Verification items for the finished model (mm, model axes). A direction names the side the tool comes from. Give positions to 0.01 mm unless a question says otherwise; leave off trailing zeros. Order: outer loops, then holes, each group sorted by start corner. A loop starts at its lowest first (then second) coordinate and runs counter-clockwise, first axis right, second up. Notation, with made-up numbers: (10, 37.5) -> (29, 37.5) arc R16 cw to (29, 58.5) -> close; hole circle Ø7 at (64, 70). An arc over 180 degrees is marked (long way). Return JSON: item names as keys, results as strings. Group by question number.
(1) Tool access check on faces 1 (the face through (5.08, 28, 3)), 2 (the face through (0, 28, 4.245)), 3 (the face through (4, 1, 2.54)). Record the directions out of +Z, -Z, +X, -X, +Y, -Y that give a thin tool (end or side, any length) a straight path to the whole face; none if there is none.
(2) Release check for a two-part mould opening along X. For faces 4 (the face through (3.726, 0, 4)), 5 (the face through (-2.961, 1, 4)), 6 (the face through (-8.69, 0, 3)), 7 (the face through (0, 28, 1.705)) record: pulls with the +X half, pulls with the -X half, needs draft (parallel to the pull), parting line crosses it, or undercut.
(3) Cross-section at C-C on x = -7.5. Enter the section's corners in (y, z), then the cut area to 3 significant figures.
(4) Thickness scan on line 1 along Y through (x, z) = (0.25, 2.8); line 2 along X through (y, z) = (7.5, 3.65); line 3 along Y through (x, z) = (-8, 4.9). Record the ranges inside material, lowest first.
(5) Cross-section at B-B on z = 1.05. Enter the section's corners in (x, y).
(6) Depth check by flat-ended pin: pin 1 Ø0.8 at (y, z) = (26, 3) entering from -X; pin 2 Ø1.5 at (x, z) = (-6.5, 2.5) entering from +Y; pin 3 Ø4 at (x, y) = (-2, 27.5) entering from -Z (3 decimals). Enter the tip coordinate at first touch or a pass-through.
(7) Cross-section at A-A on z = 3.1. State how many separate pieces and enclosed holes the cut face has, then the cut area to 3 significant figures.
from build123d import *

# Parameters (mm, degrees)
SKETCH1_W           = 17.38
SKETCH1_H           = 47.498
BOSS_EXTRUDE1_DEPTH = 5.95
CUT_EXTRUDE1_DEPTH  = 3.41
SKETCH3_W           = 10.16
SKETCH3_H           = 2.54
BOSS_EXTRUDE2_DEPTH = 7.62


with BuildPart() as part:
    # Sketch1 → Boss-Extrude1 (new body)
    with BuildSketch(Plane.XY):
        Rectangle(SKETCH1_W, SKETCH1_H)
    extrude(amount=BOSS_EXTRUDE1_DEPTH)

    # Sketch2 → Cut-Extrude1 (cut)
    with BuildSketch(Plane.XY.offset(5.95)):
        with BuildLine():
            add(Edge.make_bspline(
                [(0.550302732, -8.226542522), (0.379735674, -8.222982783), (0.040169774, -8.215896034), (-0.463839474, -8.15812923), (-0.957953156, -8.065305599), (-1.440722609, -7.93397308), (-1.914246856, -7.765779149), (-2.375520379, -7.555268135), (-2.829688826, -7.311649662), (-3.271985998, -7.033523648), (-3.695622296, -6.719710376), (-4.100608986, -6.379462985), (-4.482356898, -6.010283848), (-4.834867943, -5.609039062), (-5.170252218, -5.186152795), (-5.479691278, -4.732982281), (-5.767177385, -4.252361088), (-6.026195622, -3.745122286), (-6.262649235, -3.220813492), (-6.463385677, -2.677755241), (-6.63458604, -2.121971034), (-6.777705411, -1.554373675), (-6.884857685, -0.974513718), (-6.963012588, -0.382925268), (-7.013958172, 0.222378933), (-7.018848737, 0.631170896), (-7.021320272, 0.837761211)],
                knots=[0, 0, 0, 0, 0.935229359, 1.861860104, 2.778365642, 3.690213086, 4.602953262, 5.531139642, 6.468158725, 7.427752723, 8.393775505, 9.35721743, 10.326918663, 11.30305363, 12.284324182, 13.285316018, 14.310199044, 15.353667505, 16.407211588, 17.462763663, 18.526572315, 19.595421863, 20.671172186, 21.758519085, 22.867227609, 24, 24, 24, 24], degree=3))
            add(Edge.make_bspline(
                [(-7.021320272, 0.837761211), (-7.019018375, 1.043132905), (-7.014463737, 1.449490733), (-6.960970524, 2.051780421), (-6.891552806, 2.643471616), (-6.774881724, 3.22130983), (-6.639867653, 3.790672361), (-6.466996952, 4.345851556), (-6.265031095, 4.888970049), (-6.033789785, 5.416782083), (-5.779586146, 5.927183042), (-5.493336967, 6.408001352), (-5.191668967, 6.865492143), (-4.867252969, 7.295030074), (-4.519766848, 7.695667308), (-4.148181052, 8.065835718), (-3.757073623, 8.410721014), (-3.34206406, 8.721642737), (-2.915815576, 9.008687913), (-2.469246401, 9.247584189), (-2.017296753, 9.462224383), (-1.549212621, 9.625945007), (-1.073318626, 9.765137224), (-0.584345141, 9.855228751), (-0.084297826, 9.914279226), (0.252836758, 9.921036178), (0.42342487, 9.924455156)],
                knots=[0, 0, 0, 0, 1.133047579, 2.241899783, 3.335215261, 4.419027891, 5.492968413, 6.563480614, 7.625684211, 8.689373082, 9.742419676, 10.770259333, 11.775568516, 12.765501156, 13.738725683, 14.699866048, 15.658232057, 16.613840314, 17.560131627, 18.490982804, 19.406287858, 20.318317554, 21.224515383, 22.140052105, 23.058877329, 24, 24, 24, 24], degree=3))
            add(Edge.make_bspline(
                [(0.42342487, 9.924455156), (0.559148281, 9.921645508), (0.832560203, 9.915985532), (1.243556078, 9.86754079), (1.660769686, 9.798955016), (2.079767463, 9.691960066), (2.500803763, 9.563498986), (2.916875885, 9.402970456), (3.324320864, 9.20650682), (3.725724779, 8.983747658), (4.116057738, 8.734840571), (4.491372535, 8.460890619), (4.850047767, 8.162570258), (5.075596578, 7.946758141), (5.1888081, 7.838433835)],
                knots=[0, 0, 0, 0, 0.915509886, 1.844275157, 2.789506648, 3.766658426, 4.759580674, 5.758727315, 6.772399487, 7.809398841, 8.854855904, 9.894060884, 10.942949104, 12, 12, 12, 12], degree=3))
            add(Edge.make_bspline(
                [(5.1888081, 7.838433835), (5.389513895, 7.625274141), (5.793462123, 7.196260714), (6.305371236, 6.463621807), (6.75436753, 5.667322469), (7.122251761, 4.802237473), (7.423384955, 3.884299926), (7.633961726, 2.916595545), (7.76448607, 1.904889958), (7.778790351, 1.215067432), (7.786072571, 0.863883124)],
                knots=[0, 0, 0, 0, 0.919193343, 1.850003994, 2.80051803, 3.788248458, 4.799621584, 5.832655484, 6.896618542, 8, 8, 8, 8], degree=3))
            add(Edge.make_bspline(
                [(7.786072571, 0.863883124), (7.78352135, 0.647353624), (7.778470942, 0.218710705), (7.728707805, -0.415441181), (7.646780013, -1.034640035), (7.530912683, -1.637393561), (7.386051211, -2.223133728), (7.210848244, -2.789509257), (7.001599425, -3.333806008), (6.762418257, -3.857277855), (6.494119995, -4.359757078), (6.189400077, -4.837839702), (5.857936501, -5.297417839), (5.49711839, -5.733205631), (5.11051594, -6.138422567), (4.702735067, -6.510368516), (4.273224882, -6.842804833), (3.972375106, -7.039318089), (3.823005232, -7.136885589)],
                knots=[0, 0, 0, 0, 1.113772475, 2.204829758, 3.27005864, 4.325555321, 5.360779408, 6.372800007, 7.37346729, 8.358543946, 9.331995144, 10.301336045, 11.272892343, 12.245459715, 13.209547844, 14.151832625, 15.082397426, 16, 16, 16, 16], degree=3))
            add(Edge.make_bspline(
                [(3.823005232, -7.136885589), (3.683147268, -7.222635548), (3.409480365, -7.390426678), (2.994828528, -7.617684008), (2.579610392, -7.803303161), (2.168546265, -7.957578038), (1.759611301, -8.078012453), (1.354366193, -8.164644128), (0.950796586, -8.213781885), (0.683522897, -8.222297827), (0.550302732, -8.226542522)],
                knots=[0, 0, 0, 0, 1.125879178, 2.203062722, 3.242368383, 4.244546476, 5.214349521, 6.165371228, 7.085545794, 8, 8, 8, 8], degree=3))
        make_face()
        with BuildLine():
            Line((-2.961228686, 2.472246611), (-2.961228686, -0.774333977))
            add(Edge.make_bspline(
                [(-2.961228686, -0.774333977), (-2.959967414, -1.061739722), (-2.957525343, -1.618214071), (-2.913735758, -2.423346557), (-2.85314572, -3.170531032), (-2.764518939, -3.859438567), (-2.648829977, -4.489436798), (-2.514239059, -5.064508473), (-2.34558364, -5.578937047), (-2.157613001, -6.039786153), (-1.937036422, -6.441665454), (-1.688349536, -6.790544547), (-1.412867317, -7.087851968), (-1.105878525, -7.330815974), (-0.771392176, -7.520290022), (-0.406109176, -7.649721448), (-0.015966549, -7.736110927), (0.255015986, -7.744563056), (0.393571255, -7.748884688)],
                knots=[0, 0, 0, 0, 1.600918194, 3.099694165, 4.490651416, 5.776535035, 6.967210561, 8.058031995, 9.063903489, 9.980236553, 10.826977267, 11.611606621, 12.361723182, 13.077105204, 13.784521788, 14.492616884, 15.229264454, 16, 16, 16, 16], degree=3))
            add(Edge.make_bspline(
                [(0.393571255, -7.748884688), (0.528245131, -7.743778256), (0.791040711, -7.733813831), (1.172625546, -7.658529716), (1.52755677, -7.529237818), (1.857994163, -7.353860426), (2.162648136, -7.126013205), (2.433191301, -6.842648648), (2.682181228, -6.513316438), (2.906762463, -6.134934559), (3.098668036, -5.70286344), (3.264765351, -5.222717393), (3.41242016, -4.695082575), (3.523579553, -4.114111113), (3.619116063, -3.484551491), (3.677799548, -2.803976451), (3.722465518, -2.074804922), (3.724782967, -1.571754083), (3.725980985, -1.31169904)],
                knots=[0, 0, 0, 0, 0.799284555, 1.559682205, 2.297915387, 3.034706454, 3.773235106, 4.546189228, 5.35267469, 6.22028085, 7.152378913, 8.154412891, 9.234837652, 10.402226976, 11.66392272, 13.013895726, 14.456316111, 16, 16, 16, 16], degree=3))
            Line((3.725980985, -1.31169904), (3.725980985, 2.02071069))
            add(Edge.make_bspline(
                [(3.725980985, 2.02071069), (3.723748812, 2.257046674), (3.71936631, 2.721053283), (3.708560971, 3.40434293), (3.670819489, 4.059661491), (3.633719336, 4.679578677), (3.580286013, 5.245401301), (3.527872185, 5.741345681), (3.463618752, 6.156666795), (3.405129076, 6.40324308), (3.378932715, 6.513679687)],
                knots=[0, 0, 0, 0, 1.256484259, 2.466898997, 3.63225641, 4.745570288, 5.768126857, 6.653192896, 7.396791916, 8, 8, 8, 8], degree=3))
            add(Edge.make_bspline(
                [(3.378932715, 6.513679687), (3.320948737, 6.744215447), (3.210519313, 7.183266572), (2.967701416, 7.785371154), (2.672577177, 8.299006644), (2.320734987, 8.721868888), (1.906870016, 9.046189335), (1.444126514, 9.282221464), (0.924296657, 9.424668031), (0.55992772, 9.439245863), (0.371181044, 9.446797322)],
                knots=[0, 0, 0, 0, 1.239636621, 2.360865202, 3.376378042, 4.320723676, 5.213018588, 6.101502634, 7.016559783, 8, 8, 8, 8], degree=3))
            add(Edge.make_bspline(
                [(0.371181044, 9.446797322), (0.183805449, 9.438721037), (-0.178748844, 9.423094179), (-0.695940302, 9.287727329), (-1.154051557, 9.05336189), (-1.488973453, 8.787875802), (-1.719418951, 8.527231967), (-1.889320993, 8.311817875), (-2.042444584, 8.067599792), (-2.177811432, 7.796765191), (-2.311332426, 7.50616398), (-2.42423477, 7.187961886), (-2.529779888, 6.84706081), (-2.621917406, 6.480649791), (-2.706054572, 6.086538044), (-2.769578415, 5.66104142), (-2.830815218, 5.205995831), (-2.878464235, 4.719303951), (-2.91578194, 4.201662227), (-2.939863819, 3.652856534), (-2.961426072, 3.073215175), (-2.961295697, 2.676269351), (-2.961228686, 2.472246611)],
                knots=[0, 0, 0, 0, 1.298765628, 2.512990303, 3.674827545, 4.847513772, 5.452475075, 6.086065062, 6.74935122, 7.448024762, 8.185900438, 8.966790838, 9.788537819, 10.6614505, 11.587369526, 12.583477292, 13.645459279, 14.77306755, 15.9758581, 17.246032595, 18.584512186, 20, 20, 20, 20], degree=3))
        make_face(mode=Mode.SUBTRACT)
    extrude(amount=-CUT_EXTRUDE1_DEPTH, mode=Mode.SUBTRACT)

    # Sketch3 → Boss-Extrude2 (add)
    with BuildSketch(Plane(origin=(0, 23.749, 0), x_dir=(1, 0, 0), z_dir=(0, 1, 0))):
        with Locations((0, -2.975)):
            Rectangle(SKETCH3_W, SKETCH3_H)
    extrude(amount=BOSS_EXTRUDE2_DEPTH)


solid = part.part
Verdict:
{
 "1": {"face 1": "+Z, -Z, +X, +Y", "face 2": "+Z, +X, -X, +Y", "face 3": "+Z"},
 "2": {"face 4": "undercut", "face 5": "undercut", "face 6": "pulls with the -X half", "face 7": "needs draft"},
 "3": {"outline": "(-23.75, 0) -> (23.75, 0) -> (23.75, 5.95) -> (-23.75, 5.95) -> close", "area": "283 mm²"},
 "4": {"line 1": "-23.75 to -8.22, -7.74 to 9.44, 9.92 to 31.37", "line 2": "-8.69 to -4.69, -2.31 to 3.08, 5.5 to 8.69", "line 3": "-23.75 to 23.75"},
 "5": {"outline": "(-8.69, -23.75) -> (8.69, -23.75) -> (8.69, 23.75) -> (-8.69, 23.75) -> close"},
 "6": {"pin 1": "x = -5.08", "pin 2": "y = 23.75", "pin 3": "z = 1.705"},
 "7": {"separate pieces": "2", "enclosed holes": "1", "area": "792 mm²"}
}
